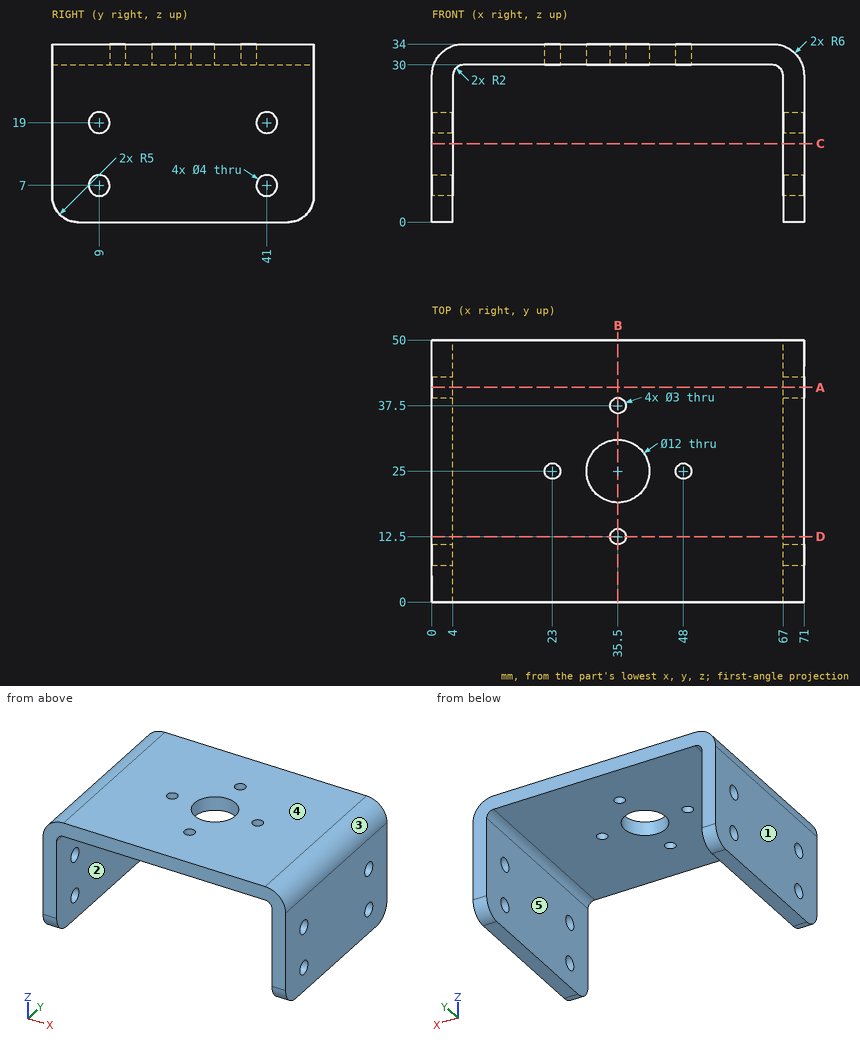
Study the drawing (mm; zero at the part's minimum x, y, z) and answer. A direction names the side the tool comes from. Round coordinates to 2 decimals unless told otherwise and drop trailing zeros. Loops run counter-clockwise (first coordinate to the right, second up) from the corner with the lowest first, then second, coordinate; pieces in that order, holes last.
Q1. Given pin 1 Ø6.5 at (y, z) = (41, 19) entering from -X; pin 2 Ø25 at (x, y) = (36.5, 20.5) entering from -Z, each flat-ended and moving along its own axis, determine where each tip first touches the part or whether it passes through.
Q2. Which of the six approach directions +Z, -Z, +X, -X, +Y, -Y give full straight-line access (tool end or side, diameter ignored) to the marked faces 4 and 5?
Q3. For a pull along X with two mould halves and no side action, classify the marked faces 1, 2 and 3 as released by +X, released by -X, zero draft, split by the parting line, or undercut.
Q4. Section A-A, the plane y = 41 is taken. Determine the outline of the cut face in (x, z), then the cut area to 3 significant figures.
Q5. Section B-B, the plane x = 35.5 is taken. Determine the outline of the cut face in (y, z), then the cut area to 3 significant figures.
Q6. Section D-D, the plane y = 12.5 is taken. Determine the outline of the cut face in (x, z).
Q7. Find the intervals of material crossed by line 1 (Y direction, x = 2, z = 7); line 2 (X direction, y = 34, z = 26); line 3 (Z direction, x = 68.5, y = 8), in increasing order.
Q8. Section C-C, the plane z = 15 is taken. Determine the outline of the cut face in (x, y), then the cut area to 3 significant figures.
Completed:
1. pin 1: stops at x = 0
1. pin 2: stops at z = 30
2. face 4: +Z, +X, -X, +Y, -Y
2. face 5: -Z, +Y, -Y
3. face 1: released by -X
3. face 2: undercut
3. face 3: released by +X
4. outline: (0, 0) - (4, 0) - (4, 5) - (0, 5) - close; (0, 9) - (4, 9) - (4, 17) - (0, 17) - close; (0, 21) - (4, 21) - (4, 28) arc R2 cw to (6, 30) - (65, 30) arc R2 cw to (67, 28) - (67, 21) - (71, 21) - (71, 28) arc R6 ccw to (65, 34) - (6, 34) arc R6 ccw to (0, 28) - close; (67, 0) - (71, 0) - (71, 5) - (67, 5) - close; (67, 9) - (71, 9) - (71, 17) - (67, 17) - close
4. area: 446 mm2
5. outline: (0, 30) - (11, 30) - (11, 34) - (0, 34) - close; (14, 30) - (19, 30) - (19, 34) - (14, 34) - close; (31, 30) - (36, 30) - (36, 34) - (31, 34) - close; (39, 30) - (50, 30) - (50, 34) - (39, 34) - close
5. area: 128 mm2
6. outline: (0, 0) - (4, 0) - (4, 28) arc R2 cw to (6, 30) - (34, 30) - (34, 34) - (6, 34) arc R6 ccw to (0, 28) - close; (37, 30) - (65, 30) arc R2 cw to (67, 28) - (67, 0) - (71, 0) - (71, 28) arc R6 ccw to (65, 34) - (37, 34) - close
7. line 1: y = 0 to 7, 11 to 39, 43 to 50
7. line 2: x = 0 to 4, 67 to 71
7. line 3: z = 0 to 5.27, 8.73 to 17.27, 20.73 to 32.87
8. outline: (0, 0) - (4, 0) - (4, 50) - (0, 50) - close; (67, 0) - (71, 0) - (71, 50) - (67, 50) - close
8. area: 400 mm2
